from build123d import *

# Parameters (mm, degrees)
SKETCH1_W                      = 60
SKETCH1_H                      = 70
BASE_FLANGE3_DEPTH             = 1.524
EDGE_FLANGE1_STRIP_W           = 10.096
EDGE_FLANGE1_STRIP_H           = 1.524
EDGE_FLANGE1_STRIP_CUT_DEPTH   = 70
EDGE_FLANGE1_STRIP_2_W         = 10.096
EDGE_FLANGE1_STRIP_2_H         = 1.524
EDGE_FLANGE1_STRIP_CUT_2_DEPTH = 70
EDGE_FLANGE1_DEPTH             = 70
EDGE_FLANGE1_BEND_DEPTH        = 70
F_7_0_7_DIAMETER_HOLE1_D       = 7
M6_CLEARANCE_HOLE1_D           = 6.6


# Sheet-metal steps are written as plain solids
with BuildPart() as part:
    # Sketch1 → Base-Flange3 (new body)
    with BuildSketch(Plane(origin=(0, 0, 0), x_dir=(1, 0, 0), z_dir=(0, 1, 0))):
        Rectangle(SKETCH1_W, SKETCH1_H)
    extrude(amount=-BASE_FLANGE3_DEPTH)

    # Edge-Flange1 strip (across the edge) → Edge-Flange1 strip cut (cut)
    with BuildSketch(Plane(origin=(-30, 0, -35), x_dir=(1, 0, 0), z_dir=(0, 0, 1))):
        with Locations((-3.048, -0.762)):
            Rectangle(EDGE_FLANGE1_STRIP_W, EDGE_FLANGE1_STRIP_H)
    extrude(amount=EDGE_FLANGE1_STRIP_CUT_DEPTH, mode=Mode.SUBTRACT)

    # Edge-Flange1 strip 2 (across the edge) → Edge-Flange1 strip cut 2 (cut)
    with BuildSketch(Plane(origin=(30, 0, 35), x_dir=(-1, 0, 0), z_dir=(0, 0, -1))):
        with Locations((-3.048, -0.762)):
            Rectangle(EDGE_FLANGE1_STRIP_2_W, EDGE_FLANGE1_STRIP_2_H)
    extrude(amount=EDGE_FLANGE1_STRIP_CUT_2_DEPTH, mode=Mode.SUBTRACT)

    # Edge-Flange1 section (across the edge) → Edge-Flange1 (add)
    with BuildSketch(Plane(origin=(-30, 0, -35), x_dir=(1, 0, 0), z_dir=(0, 0, 1))):
        with BuildLine():
            Line((-1.524, 2), (-1.524, 48.476))
            Line((-1.524, 48.476), (0, 48.476))
            Line((0, 48.476), (0, 2))
            ThreePointArc((0, 2), (0.585786438, 0.585786438), (2, 0))
            Line((2, 0), (2, -1.524))
            ThreePointArc((2, -1.524), (-0.491844297, -0.491844297), (-1.524, 2))
        make_face()
    extrude(amount=EDGE_FLANGE1_DEPTH)

    # Edge-Flange1 section 2 (across the edge) → Edge-Flange1 bend (add)
    with BuildSketch(Plane(origin=(30, 0, 35), x_dir=(-1, 0, 0), z_dir=(0, 0, -1))):
        with BuildLine():
            Line((-1.524, 2), (-1.524, 48.476))
            Line((-1.524, 48.476), (0, 48.476))
            Line((0, 48.476), (0, 2))
            ThreePointArc((0, 2), (0.585786438, 0.585786438), (2, 0))
            Line((2, 0), (2, -1.524))
            ThreePointArc((2, -1.524), (-0.491844297, -0.491844297), (-1.524, 2))
        make_face()
    extrude(amount=EDGE_FLANGE1_BEND_DEPTH)

    # Ø7.0 (7) Diameter Hole1 (through all)
    with Locations(Plane.ZY.offset(31.524)):
        with Locations((21.143083968, 25.4), (-21.143083968, 40.79090645)):
            Hole(F_7_0_7_DIAMETER_HOLE1_D / 2)

    # M6 Clearance Hole1 (through all)
    with Locations(Plane(origin=(0, 0, 0), x_dir=(1, 0, 0), z_dir=(0, 1, 0))):
        with Locations((-18, -25), (18, -25), (18, 25), (-18, 25)):
            Hole(M6_CLEARANCE_HOLE1_D / 2)


solid = part.part
For this review, take the finished solid that the model builds, in its own axes (mm). A direction names the side the tool comes from. Coordinates: 2 decimals unless noted, no trailing zeros. Loops run counter-clockwise (first coordinate to the right, second up) from the corner with the lowest first, then second, coordinate; pieces in that order, holes last. Notation, with made-up numbers: (73.5, 44.5) - (81.5, 44.5) arc R10 cw to (81.5, 58.5) - close; hole circle Ø8 at (73, -19.5). An arc over 180 degrees is marked (long way). Use a Markdown table: item, result. Add a question column.
Item 1: We need section A-A (y = 21). Give the boundary of the cut face in (x, z).
Item 2: Tool access review of faces 1 (the face through (-29.43, 0.6, -0.49)), 2 (the face through (-0.1, -0.5, 35)): name each direction out of +Z, -Z, +X, -X, +Y, -Y from which nothing blocks a thin tool from reaching the whole face with its end or side.
Item 3: We need section B-B (x = 18). Give the boundary of the cut face in (y, z), and give its area (3 significant figures).
Item 4: Insertion check: pin 1 Ø1.5 at (x, z) = (-13, -18) entering from +Y. The pin has a flat end and moves straight along its axis. Give the tip position at first contact, or say it passes through.
Item 5: We need section D-D (z = -26). Give the boundary of the cut face in (x, y), and give its area (3 significant figures).
Item 6: Mouldability with a two-part tool opening along Z and no side actions: class faces 3 (the face through (31.524, 25, 0)), 4 (the face through (-0.1, -0.5, -35)), 5 (the face through (20.619, -0.773, 27.008)) as pulls with the +Z half, pulls with the -Z half, needs draft (parallel to the pull), parting line crosses it, or undercut.
Item 7: For line 1 (Z direction, x = 18, y = -1.05); line 2 (X direction, y = 45.5, z = -21); line 3 (X direction, y = -1, z = -25), list the stretches that pass through material, from the lowest coordinate up.
Item 8: We need section C-C (z = 23.5). Give the boundary of the cut face in (x, y).
Results list:
| question | item | result |
|---|---|---|
| 1 | outline | (-31.52, -35) - (-30, -35) - (-30, 35) - (-31.52, 35) - close; (30, -35) - (31.52, -35) - (31.52, 35) - (30, 35) - close |
| 2 | face 1 | +Z, -Z, +Y |
| 2 | face 2 | +Z, +X, -X, +Y, -Y |
| 3 | outline | (-1.52, -35) - (0, -35) - (0, -28.3) - (-1.52, -28.3) - close; (-1.52, -21.7) - (0, -21.7) - (0, 21.7) - (-1.52, 21.7) - close; (-1.52, 28.3) - (0, 28.3) - (0, 35) - (-1.52, 35) - close |
| 3 | area | 86.6 mm^2 |
| 4 | pin 1 | stops at y = 0 |
| 5 | outline | (-31.52, 2) arc R3.52 ccw to (-28, -1.52) - (-21.14, -1.52) - (-21.14, 0) - (-28, 0) arc R2 cw to (-30, 2) - (-30, 48.48) - (-31.52, 48.48) - close; (-14.86, -1.52) - (14.86, -1.52) - (14.86, 0) - (-14.86, 0) - close; (21.14, -1.52) - (28, -1.52) arc R3.52 ccw to (31.52, 2) - (31.52, 48.48) - (30, 48.48) - (30, 2) arc R2 cw to (28, 0) - (21.14, 0) - close |
| 5 | area | 221 mm^2 |
| 6 | face 3 | needs draft |
| 6 | face 4 | pulls with the -Z half |
| 6 | face 5 | undercut |
| 7 | line 1 | z = -35 to -28.3, -21.7 to 21.7, 28.3 to 35 |
| 7 | line 2 | x = -31.52 to -30, 30 to 31.52 |
| 7 | line 3 | x = -29.85 to -21.3, -14.7 to 14.7, 21.3 to 29.85 |
| 8 | outline | (-31.52, 2) arc R3.52 ccw to (-28, -1.52) - (-20.94, -1.52) - (-20.94, 0) - (-28, 0) arc R2 cw to (-30, 2) - (-30, 22.81) - (-31.52, 22.81) - close; (-31.52, 27.99) - (-30, 27.99) - (-30, 48.48) - (-31.52, 48.48) - close; (-15.06, -1.52) - (15.06, -1.52) - (15.06, 0) - (-15.06, 0) - close; (20.94, -1.52) - (28, -1.52) arc R3.52 ccw to (31.52, 2) - (31.52, 22.81) - (30, 22.81) - (30, 2) arc R2 cw to (28, 0) - (20.94, 0) - close; (30, 27.99) - (31.52, 27.99) - (31.52, 48.48) - (30, 48.48) - close |
